```python
from build123d import *

# Parameters (mm, degrees)
F0_W      = 222.25
F0_H      = 120.65
F1_DEPTH  = 12.7
F3_DEPTH  = 107.95
F5_DEPTH  = 107.95
F6_SIZE2  = 5.08
F6_SIZE   = 5.08
F7_R      = 19.05
F8_DEPTH  = 192.278
F9_SIZE   = 5.08
F10_SIZE  = 5.08
F11_SIZE  = 5.08
F12_R     = 6.35
F12_R_2   = 7.9375
F13_DEPTH = 25.4
F15_DEPTH = 216.154


with BuildPart() as f1:
    # F0 (on Top) → F1 (new body)
    with BuildSketch(Plane.XY):
        with Locations((5.2343402058, -36.9766564707)):
            Rectangle(F0_W, F0_H)
    extrude(amount=F1_DEPTH)

    # F2 (on face) → F3 (join)
    with BuildSketch(Plane.XY.offset(12.7)):
        Polygon((-58.2656597942, 23.3483435293), (-58.2656597942, -85.1823836565), (-58.2656597942, -97.3016564707), (-39.2156597942, -97.3016564707), (-39.2156597942, 23.3483435293), align=None)
    extrude(amount=F3_DEPTH)

    # F4 (on face) → F5 (join)
    with BuildSketch(Plane.XY.offset(12.7)):
        Polygon((30.6343402058, 23.3483435293), (30.6343402058, -84.2409580946), (30.6343402058, -97.3016564707), (49.6843402058, -97.3016564707), (49.6843402058, 23.3483435293), align=None)
    extrude(amount=F5_DEPTH)

    # F6
    f6_edges = [f1.edges().sort_by_distance(p)[0] for p in [
        (40.15934, 23.348344, 120.65),
    ]]
    chamfer(f6_edges, length=F6_SIZE, length2=F6_SIZE2)

    # F7 (on face) → F8 (cut)
    with BuildSketch(Plane.YZ.offset(49.6843402058)):
        with Locations((-24.1999551654, 82.55)):
            Circle(F7_R)
    extrude(amount=-F8_DEPTH, mode=Mode.SUBTRACT)

    # F9
    f9_edges = [f1.edges().sort_by_distance(p)[0] for p in [
        (-48.74066, 23.348344, 120.65),
    ]]
    chamfer(f9_edges, length=F9_SIZE)

    # F10
    f10_edges = [f1.edges().sort_by_distance(p)[0] for p in [
        (116.35934, -97.301656, 6.35),
    ]]
    chamfer(f10_edges, length=F10_SIZE)

    # F11
    f11_edges = [f1.edges().sort_by_distance(p)[0] for p in [
        (116.35934, 23.348344, 6.35),
    ]]
    chamfer(f11_edges, length=F11_SIZE)

    # F12 (on face) → F13 (cut)
    with BuildSketch(Plane.XY.offset(12.7)):
        with Locations((99.7244338119, -78.2516564707)):
            Circle(F12_R)
        with Locations((99.9952717069, -2.0516564707)):
            Circle(F12_R)
        with Locations((-80.1142602397, -78.2516564707)):
            Circle(F12_R)
        with Locations((0, -87.7766564707)):
            Circle(F12_R_2)
    extrude(amount=-F13_DEPTH, mode=Mode.SUBTRACT)

    # F14 (on face) → F15 (cut)
    with BuildSketch(Plane.YZ.offset(49.6843402058)):
        Polygon((-97.3016564707, 120.65), (-97.3016564707, 33.7335392833), (-32.7723734081, 120.65), align=None)
    extrude(amount=-F15_DEPTH, mode=Mode.SUBTRACT)


solid = f1.part
```
Design review of the part built by this model. Coordinates are the model's own, in mm. A direction names the side the tool comes from. Give positions to 0.01 mm unless a question says otherwise; leave off trailing zeros. Loops run counter-clockwise (first coordinate to the right, second up) from the corner with the lowest first, then second, coordinate; pieces in that order, holes last. Notation, with made-up numbers: (84.5, 5) -> (108.5, 5) arc R25 ccw to (108.5, 21) -> close; hole circle Ø8 at (-9.5, -14). An arc over 180 degrees is marked (long way). Write each question's results on one line, items separated by ' | '.
Q1. Take a section at A-A, the plane x = 0. Write out the cut boundary in (y, z), plus the area to 3 significant figures.
Reply:
outline: (-97.3, 0) -> (-95.71, 0) -> (-95.71, 12.7) -> (-97.3, 12.7) -> close; (-79.84, 0) -> (23.35, 0) -> (23.35, 12.7) -> (-79.84, 12.7) -> close | area: 1,330 mm²
Q2. Wall thickness on L1, parallel to X at y = 12.5, z = 107; L2, parallel to Z at x = 15, y = 18.5; L3, parallel to X at y = -75.5, z = 7.5: over which ranges is each line inside the solid? List them lowest first.
Reply:
L1: x = -58.27 to -39.22, 30.63 to 49.68 | L2: z = 0 to 12.7 | L3: x = -105.89 to -85.84, -74.39 to 94, 105.45 to 116.36
Q3. The part is to be moulded in two halves that separate along Y. For faces 1 (the face through (98.35, -84.45, 6.44)), 2 (the face through (113.784, 20.844, 6.261)), 3 (the face through (4, -36, 0)), 4 (the face through (-1.721, -95.525, 6.439)), say which applies: +Y half, -Y half, draft (parallel to the pull), parting line (faces both ways), or undercut.
Reply:
face 1: undercut | face 2: +Y half | face 3: draft | face 4: undercut
Q4. For pin 1 Ø1.5 at (x, y) = (-3, -44) entering from -Z; pin 2 Ø10 at (x, y) = (-43, -79) entering from +Z; pin 3 Ø14.5 at (x, y) = (-75, -59.5) entering from +Z; pin 4 Ø3 at (x, z) = (-38.5, 78) entering from -Y, all flat-tipped, find the tip position at first contact; note any pin that passes through.
Reply:
pin 1: stops at z = 0 | pin 2: stops at z = 65.12 | pin 3: stops at z = 12.7 | pin 4: stops at y = -65.42
Q5. Machinability: for faces 5 (the face through (-5, -36, 12.7)), 6 (the face through (-48.61, 20.77, 118.15)), 7 (the face through (-58.266, -23, 54)), which of the approach directions +Z, -Z, +X, -X, +Y, -Y give a long, thin tool a straight path to every point of the face, cutting with its end or side? Answer none if there is none.
Reply:
face 5: +Z, +Y, -Y | face 6: +Z, +X, -X, +Y | face 7: +Z, -X, +Y, -Y
Q6. Take a section at D-D, the plane x = -42.5. Write out the cut boundary in (y, z).
Reply:
outline: (-97.3, 0) -> (23.35, 0) -> (23.35, 115.57) -> (18.27, 120.65) -> (-32.77, 120.65) -> (-97.3, 33.73) -> close; hole circle Ø38.1 at (-24.2, 82.55)
Q7. Take a section at B-B, the plane z = 23. Write out the cut boundary in (x, y), plus the area to 3 significant figures.
Reply:
outline: (-58.27, -97.3) -> (-39.22, -97.3) -> (-39.22, 23.35) -> (-58.27, 23.35) -> close; (30.63, -97.3) -> (49.68, -97.3) -> (49.68, 23.35) -> (30.63, 23.35) -> close | area: 4,600 mm²
Q8. Take a section at C-C, the plane z = 67. Write out the cut boundary in (x, y).
Reply:
outline: (-58.27, -72.6) -> (-39.22, -72.6) -> (-39.22, -35.2) -> (-58.27, -35.2) -> close; (-58.27, -13.2) -> (-39.22, -13.2) -> (-39.22, 23.35) -> (-58.27, 23.35) -> close; (30.63, -72.6) -> (49.68, -72.6) -> (49.68, -35.2) -> (30.63, -35.2) -> close; (30.63, -13.2) -> (49.68, -13.2) -> (49.68, 23.35) -> (30.63, 23.35) -> close
